Build history of the part. All positions in model axes, mm. Give positions to 0.01 mm unless a question says otherwise; leave off trailing zeros. Order: outer loops, then holes, each group sorted by start corner. A loop starts at its lowest first (then second) coordinate and runs counter-clockwise, first axis right, second up. Notation, with made-up numbers: (-9, 52.25) - (22, 52.25) arc R13 ccw to (22, 60.25) - close; hole circle Ø4 at (19, 61.25). An arc over 180 degrees is marked (long way). Use a Markdown table: item, result.
from build123d import *


with BuildPart() as f2:
    # F2: sweep along a path in F1
    with BuildLine(Plane.XY) as f2_path:
        ThreePointArc((69.70714, 53.368706), (8.386043, 54.585932), (-19.580629, 0))
    # F0 (on Front) → F2 (sweep)
    with BuildSketch(Plane.XZ):
        with BuildLine():
            Line((-19.510009, 0), (-49.763733, 0))
            ThreePointArc((-49.763733, 0), (-53.299267, -1.464466), (-54.763733, -5))
            Line((-54.763733, -5), (-54.763733, -25.508031))
            ThreePointArc((-54.763733, -25.508031), (-53.299267, -29.043565), (-49.763733, -30.508031))
            Line((-49.763733, -30.508031), (-19.510009, -30.508031))
            Line((-19.510009, -30.508031), (-19.510009, 0))
        make_face()
    sweep(path=f2_path.line)


solid = f2.part
1) Two-plate mould, pull along X, no slides. Class faces 1 (the cylindrical face through (9.2, 54.98, -15.04)), 2 (the flat face through (80.67, 67.39, -15.04)), 3 (the flat face through (8, 61, 0)): +X half, -X half, draft (parallel to the pull), parting line (faces both ways), or undercut.
Computed:
| item | result |
|---|---|
| face 1 | undercut |
| face 2 | +X half |
| face 3 | draft |
2) Pin check, flat tips, straight feed: P1, Ø10, axis at x = 45.5, z = -21.5, coming from the -Y side; P2, Ø6, axis at y = 81, z = -5.5, coming from the +X side; P3, Ø2, axis at x = -15, y = 82, coming from the -Z side; P4, Ø6, axis at x = -30.5, z = -14, coming from the +Y side. Stop position of each tip, or through.
Computed:
| item | result |
|---|---|
| P1 | stops at y = 61.36 |
| P2 | stops at x = 91.38 |
| P3 | stops at z = -27.42 |
| P4 | stops at y = 70.82 |
3) Wall check: line 1 (X direction, y = 9.5, z = -18); line 2 (X direction, y = 6.5, z = -24); line 3 (X direction, y = 58, z = -14). Give the ranges that are in metal, low to high. Write a range as from..to.
Computed:
| item | result |
|---|---|
| line 1 | x = -54.78..-19.54 |
| line 2 | x = -54.88..-19.7 |
| line 3 | x = -38.25..15.22, 60.93..73.33 |
4) Slice it at A-A (z = -17). Write the cut outline in (x, y).
Computed:
| item | result |
|---|---|
| outline | (-54.76, 0) - (-19.51, 0) arc R57.79 cw to (69.66, 53.31) - (91.38, 81.09) arc R92.97 ccw to start |
